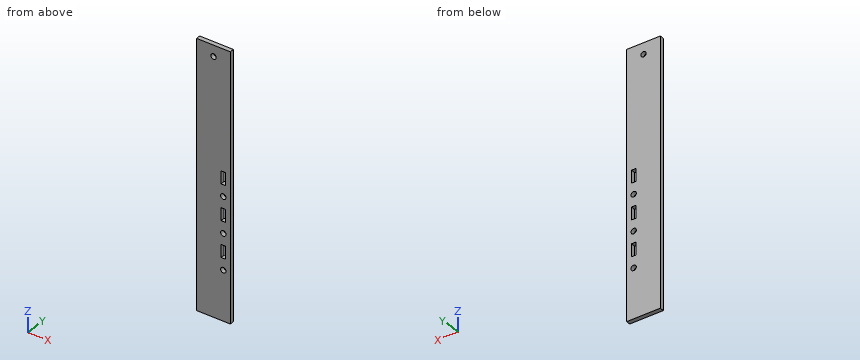
```python
from build123d import *

# Parameters (mm, degrees)
SKETCH1_W           = 19.05
SKETCH1_H           = 2.38125
BOSS_EXTRUDE1_DEPTH = 88.9
SKETCH5_R           = 1.524
CUT_EXTRUDE4_DEPTH  = 3.38125
SKETCH9_W           = 19.05
SKETCH9_H           = 29.6545
BOSS_EXTRUDE4_DEPTH = 2.38125
SKETCH10_W          = 2.47269
SKETCH10_H          = 3.58775
SKETCH10_R          = 1.524
CUT_EXTRUDE5_DEPTH  = 3.38125
BOSS_EXTRUDE5_DEPTH = 2.38125
SKETCH11_R          = 1.524
CUT_EXTRUDE6_DEPTH  = 3.38125


with BuildPart() as part:
    # Sketch1 → Boss-Extrude1 (new body)
    with BuildSketch(Plane.XY):
        with Locations((9.525, 1.190625)):
            Rectangle(SKETCH1_W, SKETCH1_H)
    extrude(amount=BOSS_EXTRUDE1_DEPTH)

    # Sketch5 → Cut-Extrude4 (cut, through all)
    with BuildSketch(Plane(origin=(0, 2.38125, 0), x_dir=(1, 0, 0), z_dir=(0, 1, 0))):
        with Locations((15.08125, -39.14775)):
            Circle(SKETCH5_R)
        with Locations((15.08125, -18.82775)):
            Circle(SKETCH5_R)
        Polygon((16.317595, -28.98775), (16.317595, -32.5755), (15.08125, -32.5755), (13.844905, -32.5755), (13.844905, -25.4), (16.317595, -25.4), align=None)
        Polygon((15.08125, -52.8955), (16.317595, -52.8955), (16.317595, -45.72), (13.844905, -45.72), (13.844905, -52.8955), align=None)
    extrude(amount=-CUT_EXTRUDE4_DEPTH, mode=Mode.SUBTRACT)

    # Sketch9 → Boss-Extrude4 (add)
    with BuildSketch(Plane(origin=(0, 2.38125, 0), x_dir=(1, 0, 0), z_dir=(0, 1, 0))):
        with Locations((9.525, 14.82725)):
            Rectangle(SKETCH9_W, SKETCH9_H)
    extrude(amount=-BOSS_EXTRUDE4_DEPTH)

    # Sketch10 → Cut-Extrude5 (cut, through all)
    with BuildSketch(Plane(origin=(0, 2.38125, 0), x_dir=(1, 0, 0), z_dir=(0, 1, 0))):
        with Locations((15.08125, -6.873875)):
            Rectangle(SKETCH10_W, SKETCH10_H)
        with Locations((15.08125, -10.461625)):
            Rectangle(SKETCH10_W, SKETCH10_H)
        with Locations((15.08125, 1.49225)):
            Circle(SKETCH10_R)
    extrude(amount=-CUT_EXTRUDE5_DEPTH, mode=Mode.SUBTRACT)

    # Sketch8 → Boss-Extrude5 (add)
    with BuildSketch(Plane(origin=(0, 2.38125, 0), x_dir=(1, 0, 0), z_dir=(0, 1, 0))):
        Polygon((19.05, -88.9), (0, -88.9), (0, -114.3), (0, -120.65), (19.05, -120.65), (19.05, -114.3), align=None)
    extrude(amount=-BOSS_EXTRUDE5_DEPTH)

    # Sketch11 → Cut-Extrude6 (cut, through all)
    with BuildSketch(Plane(origin=(0, 2.38125, 0), x_dir=(1, 0, 0), z_dir=(0, 1, 0))):
        with Locations((9.525, -114.3)):
            Circle(SKETCH11_R)
    extrude(amount=-CUT_EXTRUDE6_DEPTH, mode=Mode.SUBTRACT)


solid = part.part
```
Input: part model. Units: mm. Frame: model coordinates. Give positions to 0.01 mm unless a question says otherwise; leave off trailing zeros. Loops run counter-clockwise (first coordinate to the right, second up) from the corner with the lowest first, then second, coordinate; pieces in that order, holes last. Notation, with made-up numbers: (-39, -24) -> (-34, -24) arc R23 cw to (-34, -13) -> close; hole circle Ø7 at (4, 81.25). An arc over 180 degrees is marked (long way). Use a Markdown table: item, result.
Q1. Section query A-A, the plane z = 114.3. Return the cut outline in (x, y).
Entries:
| item | result |
|---|---|
| outline | (0, 0) -> (8, 0) -> (8, 2.38) -> (0, 2.38) -> close; (11.05, 0) -> (19.05, 0) -> (19.05, 2.38) -> (11.05, 2.38) -> close |
Q2. Section query B-B, the plane y = 1.2. State how many separate pieces and enclosed holes the cut face has, plus the area to 3 significant figures.
Entries:
| item | result |
|---|---|
| separate pieces | 1 |
| enclosed holes | 7 |
| area | 2,780 mm² |
Q3. First-contact query: P1, Ø1.2, axis at y = 1.5, z = 7.5, coming from the -X side. Flat tip, straight axial feed; report the tip coordinate or a pass-through.
Entries:
| item | result |
|---|---|
| P1 | stops at x = 0 |
Q4. Ray query, probe 1 along X at (y, z) = (0.85, 48.5); probe 2 along X at (y, z) = (1.5, 114.3); probe 3 along Z at (x, y) = (8.5, 2.1). Return the intervals inside material, ascending. Write a range as from..to.
Entries:
| item | result |
|---|---|
| probe 1 | x = 0..13.84, 16.32..19.05 |
| probe 2 | x = 0..8, 11.05..19.05 |
| probe 3 | z = -29.65..113.17, 115.43..120.65 |
